from build123d import *

# Parameters (mm, degrees)
BOSS_EXTRUDE1_DEPTH = 152.4
SKETCH5_R           = 3.175
CUT_EXTRUDE3_DEPTH  = 4.175
SKETCH6_R           = 3.175
CUT_EXTRUDE4_DEPTH  = 4.175


with BuildPart() as part:
    # Sketch1 → Boss-Extrude1 (new body)
    with BuildSketch(Plane(origin=(0, 0, 0), x_dir=(0, 0, -1), z_dir=(1, 0, 0))):
        Polygon((0, 0), (0, 38.1), (3.175, 38.1), (3.175, 3.175), (38.1, 3.175), (38.1, 0), align=None)
    extrude(amount=BOSS_EXTRUDE1_DEPTH)

    # Sketch5 → Cut-Extrude3 (cut, through all)
    with BuildSketch(Plane(origin=(0, 0, -3.175), x_dir=(-1, 0, 0), z_dir=(0, 0, -1))):
        with Locations((-127, 20.6375)):
            Circle(SKETCH5_R)
        with Locations((-25.4, 20.6375)):
            Circle(SKETCH5_R)
    extrude(amount=-CUT_EXTRUDE3_DEPTH, mode=Mode.SUBTRACT)

    # Sketch6 → Cut-Extrude4 (cut, through all)
    with BuildSketch(Plane(origin=(0, 3.175, 0), x_dir=(1, 0, 0), z_dir=(0, 1, 0))):
        with Locations((25.4, 20.6375)):
            Circle(SKETCH6_R)
        with Locations((127, 20.6375)):
            Circle(SKETCH6_R)
    extrude(amount=-CUT_EXTRUDE4_DEPTH, mode=Mode.SUBTRACT)


solid = part.part
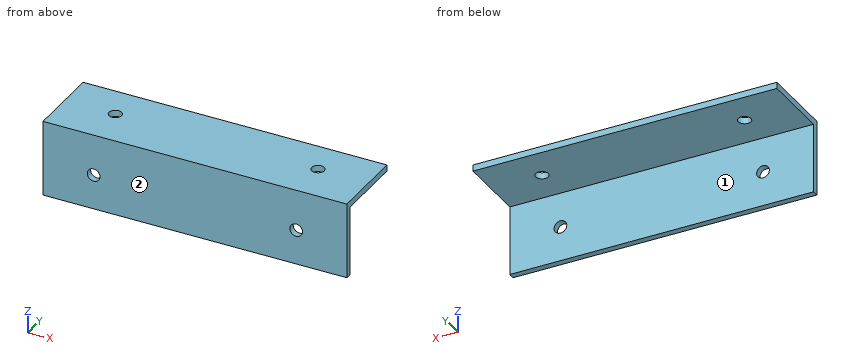
Source: CAD feature listing. Evaluate the final solid. Frame: model axes, mm. Face numbers are marked on the shaded views. A direction names the side the tool comes from. Round coordinates to 2 decimals unless told otherwise and drop trailing zeros. Loops run counter-clockwise (first coordinate to the right, second up) from the corner with the lowest first, then second, coordinate; pieces in that order, holes last. Notation, with made-up numbers: M 68,-24.5 L 104,-24.5 A21 cw 104,0.5 Z; hole C 54,50.25 d4. An arc over 180 degrees is marked long. Return JSON: item names as keys, results as strings. Group by question number.
1. Section query A-A on x = 25.4. Output: boundary loops of the cut face in (y, z) (1 decimal), and give its area (3 significant figures).
2. Section query B-B on y = 28. Output: boundary loops of the cut face in (x, z) (3 decimals), and give its area (3 significant figures).
3. Pin query (flat end, axial travel): pin 1 (10.5 mm diameter, centred on x = 82.5, z = -27.5, fed in from +Y) (3 decimals); pin 2 (8.5 mm diameter, centred on x = 127, y = 20.64, fed in from -Z) (3 decimals); pin 3 (2 mm diameter, centred on y = 5, z = -5.5, fed in from -X). Return the tip coordinate at first contact, or that it passes through.
4. Material intervals for line 1 along Y through (x, z) = (127, -1.55); line 2 along Z through (x, y) = (25.4, 1.05); line 3 along Z through (x, y) = (128.5, 24) (3 decimals), sorted ascending. Write a range as from..to.
5. Section query D-D on x = 120.5. Output: boundary loops of the cut face in (y, z) (3 decimals).
6. Reachability of the marked faces 1 and 2 from +Z, -Z, +X, -X, +Y, -Y: full face, straight path, thin tool, end or side. Return the list, or none.
7. Section query C-C on z = -7.5. Output: boundary loops of the cut face in (x, y) (3 decimals), and give its area (3 significant figures).
Checks:
{
 "1": {"outline": "M 0,-38.1 L 3.2,-38.1 L 3.2,-23.8 L 0,-23.8 Z; M 0,-17.5 L 3.2,-17.5 L 3.2,-3.2 L 17.5,-3.2 L 17.5,0 L 0,0 Z; M 23.8,-3.2 L 38.1,-3.2 L 38.1,0 L 23.8,0 Z", "area": "192 mm²"},
 "2": {"outline": "M 0,-3.175 L 152.4,-3.175 L 152.4,0 L 0,0 Z", "area": "484 mm²"},
 "3": {"pin 1": "stops at y = 3.175", "pin 2": "stops at z = -3.175", "pin 3": "passes through"},
 "4": {"line 1": "y = 0..17.46, 23.81..38.1", "line 2": "z = -38.1..-23.81, -17.46..0", "line 3": "z = -3.175..0"},
 "5": {"outline": "M 0,-38.1 L 3.175,-38.1 L 3.175,-3.175 L 38.1,-3.175 L 38.1,0 L 0,0 Z"},
 "6": {"face 1": "-Z, +X, -X, +Y", "face 2": "+Z, -Z, +X, -X, -Y"},
 "7": {"outline": "M 0,0 L 152.4,0 L 152.4,3.175 L 0,3.175 Z", "area": "484 mm²"}
}
